Autodesk Inventor part; units mm, degrees
ref_plane "Work Plane2" through (-15, 0, 0) normal (1, 0, 0) x (0, 0, -1)
ref_plane "YZ Plane" through (0, 0, 0) normal (1, 0, 0) x (0, 1, 0)
ref_plane "XZ Plane" through (0, 0, 0) normal (0, 1, 0) x (-1, 0, 0)
sketch "Sketch1" plane through (0, 0, 0) normal (0, 1, 0) x (-1, 0, 0)
  arc A0 (0.5, -14.9917) -> (-0.5, -14.9917) centre (0, 0) ccw
  arc A1 (0.5, -5.2261) -> (-0.5, -5.2261) centre (0, 0) ccw
  line L0 (-0.5, -5.2261) -> (-0.5, -14.9917)
  line L1 (0.5, -14.9917) -> (0.5, -5.2261)
  line L2 (0, 0) -> (0, -14.3069)
  dimension "d0" = 30
  dimension "d1" = 10.5
  dimension "d2" = 1
extrude "Extrusion1" add sketch "Sketch1" along normal mid plane 29
ref_plane "Work Plane2" through (-15, 0, 0) normal (1, 0, 0) x (0, 0, -1)
sketch "Sketch3" plane through (-15, 0, 0) normal (1, 0, 0) x (0, 0, -1)
  line L0 (14.9917, -14.5) -> (5.2261, -14.5)
  line L1 (14.9917, 14.5) -> (14.9917, -14.5)
  point P0 (0, 0)
  point P1 (10.9917, -7)
  dimension "d6" = 7.5
  dimension "d7" = 4
hole "Hole1" at (-15, -7, -10.9917) direction (1, 0, 0) diameter 2.8 end through all counterbore diameter 6 counterbore depth 9
mirror "Mirror1" about plane through (0, 0, 0) normal (0, 1, 0) of "Hole1"
sketch "Sketch5" plane through (0, 0, 0) normal (0, 1, 0) x (-1, 0, 0)
  arc A0 (0.5, -14.9917) -> (-0.5, -14.9917) centre (0, 0) ccw
  line L0 (13.5185, 6.5) -> (18.25, 6.5)
  line L1 (18.25, 6.5) -> (18.25, -6.5)
  line L2 (18.25, -6.5) -> (13.5185, -6.5)
  line L3 (0, 0) -> (15.3886, 0)
  line L4 (0, 0) -> (0, -14.2024)
  arc A1 (13.5185, -6.5) -> (13.5185, 6.5) centre (0, 0) ccw
  line L5 (-13.5185, 6.5) -> (-18.25, 6.5)
  line L6 (-18.25, 6.5) -> (-18.25, -6.5)
  line L7 (-18.25, -6.5) -> (-13.5185, -6.5)
  arc A2 (-13.5185, 6.5) -> (-13.5185, -6.5) centre (0, 0) ccw
  arc A3 (0.5, -5.2261) -> (-0.5, -5.2261) centre (0, 0) ccw construction
  line L8 (5.25, 0) -> (5.25, -22.9648) construction
  point P0 (-15.3886, 0)
  dimension "d23" = 13
  dimension "d36" = 13
extrude "Extrusion2" add sketch "Sketch5" along normal mid plane 15
sketch "Sketch6" plane through (-18.25, -7.5, 6.5) normal (-1, 0, 0) x (0, 0, 1)
  point P0 (-6.5, 7.5)
  point P1 (-6.5, 7.5)
hole "Hole3" at (-18.25, 0, 0) direction (1, 0, 0) diameter 8.8 end through all
fillet "Fillet1" radius 2 8 edges at (-13.5185, 0, -6.5) (-15, 7.5, 0) (-13.5185, 0, 6.5) (-15, -7.5, 0) (13.5185, 0, 6.5) (15, -7.5, 0) (13.5185, 0, -6.5) (15, 7.5, 0)
fillet "Fillet2" radius 1 8 edges at (18.25, 0, 6.5) (18.25, 7.5, 0) (18.25, 0, -6.5) (18.25, -7.5, 0) (-18.25, 0, 6.5) (-18.25, 7.5, 0) (-18.25, 0, -6.5) (-18.25, -7.5, 0)
properties part number "Space" material "ABS Plastic"
Model file for the job. Use its own axes, mm. A direction names the side the tool comes from. Give positions to 0.01 mm unless a question says otherwise; leave off trailing zeros. Loops run counter-clockwise (first coordinate to the right, second up) from the corner with the lowest first, then second, coordinate; pieces in that order, holes last. Notation, with made-up numbers: (-9.5, -18) -> (-2.5, -18) arc R32 cw to (-2.5, 18) -> close; hole circle Ø8 at (83, 71.25). An arc over 180 degrees is marked (long way). Use a Markdown table: item, result. Add a question column.
(1) Slice it at C-C on x = 9. List the corners of the cut face in (y, z), and give its area (3 significant figures).
(2) Wall check: line 1 along Z through (x, y) = (-3.5, 6.5); line 2 along X through (y, z) = (13.25, -6); line 3 along Z through (x, y) = (-14, 0.25). Give the ranges that are in metal, low to high.
(3) Drop flat-ended pins along their axis: pin 1 Ø0.8 at (x, z) = (16.5, -2.5) entering from +Y; pin 2 Ø5 at (y, z) = (-6, 8.5) entering from +X; pin 3 Ø2 at (x, y) = (-13.5, 10.5) entering from -Z; pin 4 Ø10 at (y, z) = (0, 0) entering from +X. Give the stop position or say it passes through.
(4) Tool access for faces 1 (the flat face through (-16, 0, 6.5)), 2 (the flat face through (0.5, 0, -10)), 3 (the flat face through (16, 0, -6.5)), 4 (the flat face through (-17, 7.5, 3)), 5 (the flat face through (16, 0, 6.5)): list every direction of +Z, -Z, +X, -X, +Y, -Y with a clear straight run to the whole face (end or side of a thin tool).
(5) Slice it at B-B on y = 0. List the corners of the cut face in (x, z).
(6) Slice it at A-A on z = 0. Give the number of separate pieces and of enclosed holes in the cut face, and give its area (3 significant figures).
(7) Mould opens along X. For faces 6 (the flat face through (-6, -7.7, -9.6)), 7 (the flat face through (-0.5, 0, -10)), 8 (the cylindrical face through (17.965, -7.199, -0.091)) say: +X half, -X half, draft (parallel to the pull), parting line (faces both ways), or undercut.
Filled sheet:
| question | item | result |
|---|---|---|
| 1 | outline | (-14.5, -12) -> (-7.97, -12) arc R1.4 cw (long way) to (-6.03, -12) -> (6.03, -12) arc R1.4 cw (long way) to (7.97, -12) -> (14.5, -12) -> (14.5, 12) -> (-14.5, 12) -> close; hole circle Ø8.8 at (0, 0) |
| 1 | area | 624 mm2 |
| 2 | line 1 | -14.59 to -12.3, -9.68 to -3.91, 3.91 to 14.59 |
| 2 | line 2 | -13.75 to -0.5, 0.5 to 13.75 |
| 2 | line 3 | -6.64 to -4.39, 4.39 to 6.64 |
| 3 | pin 1 | y = 7.63 |
| 3 | pin 2 | x = 18.12 |
| 3 | pin 3 | z = -8.29 |
| 3 | pin 4 | x = 18.25 |
| 4 | face 1 | +Z, -X, +Y, -Y |
| 4 | face 2 | -Z, +Y, -Y |
| 4 | face 3 | -Z, +X, +Y, -Y |
| 4 | face 4 | -X, +Y |
| 4 | face 5 | +Z, +X, +Y, -Y |
| 5 | outline | (-18.25, -5.5) arc R1 ccw to (-17.25, -6.5) -> (-14.72, -6.5) arc R2 cw to (-12.99, -7.5) arc R15 ccw to (-0.5, -14.99) -> (-0.5, -5.23) arc R5.25 cw to (-2.86, -4.4) -> (-18.25, -4.4) -> close; (-18.25, 4.4) -> (-2.86, 4.4) arc R5.25 cw to (2.86, 4.4) -> (18.25, 4.4) -> (18.25, 5.5) arc R1 ccw to (17.25, 6.5) -> (14.72, 6.5) arc R2 cw to (12.99, 7.5) arc R15 ccw to (-12.99, 7.5) arc R2 cw to (-14.72, 6.5) -> (-17.25, 6.5) arc R1 ccw to (-18.25, 5.5) -> close; (0.5, -14.99) arc R15 ccw to (12.99, -7.5) arc R2 cw to (14.72, -6.5) -> (17.25, -6.5) arc R1 ccw to (18.25, -5.5) -> (18.25, -4.4) -> (2.86, -4.4) arc R5.25 cw to (0.5, -5.23) -> close |
| 6 | separate pieces | 4 |
| 6 | enclosed holes | 0 |
| 6 | area | 437 mm2 |
| 7 | face 6 | -X half |
| 7 | face 7 | undercut |
| 7 | face 8 | +X half |
